Could you check a few things on this model? Use its own coordinates, in mm. A direction names the side the tool comes from. Coordinates: 2 decimals unless noted, no trailing zeros. Loops run counter-clockwise (first coordinate to the right, second up) from the corner with the lowest first, then second, coordinate; pieces in that order, holes last.
1) If I drill on line 1 along Z through (x, y) = (-5, 3.5); line 2 along X through (y, z) = (0.75, 0); line 3 along X through (y, z) = (1, 0.5), over which ranges is the centre line in solid material (lowest first)?
2) Imagine slicing it at C-C on z = 2.25. Please give me the cut outline in (x, y), plus the area to 3 significant figures.
3) For faces 1 (the face through (10, 4, 0)), 2 (the face through (11.5, 5, -9)), 3 (the face through (-11.5, 5, -9)), 4 (the face through (9.75, 2, 0)), which set-ups out of +Z, -Z, +X, -X, +Y, -Y let a thin tool reach every point of the face, with its end or its side?
4) Will these pins go through, and if not, where does the flat tip stop? P1, Ø3, axis at x = 16, z = 0, coming from the +Y side; P2, Ø6, axis at x = -0.5, z = -3.5, coming from the -Y side; P3, Ø1.2, axis at y = 3, z = 0.5, coming from the -X side; P4, Ø2, axis at y = 7.5, z = 3.5, coming from the +X side.
5) Imagine slicing it at A-A on z = 0. Give the number of separate pieces and of enclosed holes in the cut face, plus the area to 3 significant figures.
6) Imagine slicing it at D-D on y = 3.25. Please give me the cut outline in (x, z), plus the area to 4 significant figures.
7) Thinking about a two-plate mould opening in X: for faces 5 (the face through (0, 4, 7.5)), 6 (the face through (-19.5, 1, -9)), 7 (the face through (0, 8, 8)), which applies, released by +X, released by -X, zero draft, split by the parting line, or undercut?
8) Imagine slicing it at B-B on x = -4. Please give me the cut outline in (y, z), plus the area to 3 significant figures.
```python
from build123d import *

# Parameters (mm, degrees)
SKETCH_1_W          = 40
SKETCH_1_H          = 19
EXTRUDE_1_DEPTH     = 8
SKETCH_2_W          = 42
SKETCH_2_H          = 21
SKETCH_2_W_2        = 24
SKETCH_2_H_2        = 19
CUT_EXTRUDE_1_DEPTH = 6
SKETCH_3_W          = 19.5
SKETCH_3_H          = 15
CUT_EXTRUDE_2_DEPTH = 6
SKETCH_5_W          = 17
SKETCH_5_H          = 15
CUT_EXTRUDE_3_DEPTH = 8
SKETCH_6_W          = 15
SKETCH_6_H          = 2.2
CUT_EXTRUDE_4_DEPTH = 1.2
CHAMFER_1_SIZE      = 1.8
CHAMFER_2_SIZE      = 1
CHAMFER_3_SIZE      = 1
SKETCH_7_R          = 1.35
CUT_EXTRUDE_5_DEPTH = 23.940139494


with BuildPart() as part:
    # Эскиз1 → Бобышка-Вытянуть1 (new body)
    with BuildSketch(Plane(origin=(0, 0, 0), x_dir=(1, 0, 0), z_dir=(0, 1, 0))):
        Rectangle(SKETCH_1_W, SKETCH_1_H)
    extrude(amount=EXTRUDE_1_DEPTH)

    # Эскиз2 → Вырез-Вытянуть1 (cut)
    with BuildSketch(Plane(origin=(0, 8, 0), x_dir=(1, 0, 0), z_dir=(0, 1, 0))):
        Rectangle(SKETCH_2_W, SKETCH_2_H)
        Rectangle(SKETCH_2_W_2, SKETCH_2_H_2, mode=Mode.SUBTRACT)
    extrude(amount=-CUT_EXTRUDE_1_DEPTH, mode=Mode.SUBTRACT)

    # Эскиз3 → Вырез-Вытянуть2 (cut)
    with BuildSketch(Plane(origin=(0, 8, 0), x_dir=(1, 0, 0), z_dir=(0, 1, 0))):
        Rectangle(SKETCH_3_W, SKETCH_3_H)
    extrude(amount=-CUT_EXTRUDE_2_DEPTH, mode=Mode.SUBTRACT)

    # Эскиз5 → Вырез-Вытянуть3 (cut)
    with BuildSketch(Plane(origin=(0, 2, 0), x_dir=(1, 0, 0), z_dir=(0, 1, 0))):
        with Locations((1.25, 0)):
            Rectangle(SKETCH_5_W, SKETCH_5_H)
    extrude(amount=-CUT_EXTRUDE_3_DEPTH, mode=Mode.SUBTRACT)

    # Эскиз6 → Вырез-Вытянуть4 (cut)
    with BuildSketch(Plane(origin=(-9.75, 0, 0), x_dir=(0, 0, -1), z_dir=(1, 0, 0))):
        with Locations((0, 5.1)):
            Rectangle(SKETCH_6_W, SKETCH_6_H)
    cut_extrude_4 = extrude(amount=-CUT_EXTRUDE_4_DEPTH, mode=Mode.SUBTRACT)

    # Зеркальное отражение1: Вырез-Вытянуть4 across plane
    add(cut_extrude_4.mirror(Plane(origin=(0, 0, 0), x_dir=(0, 0, 1), z_dir=(1, 0, 0))), mode=Mode.SUBTRACT)

    # Фаска1
    chamfer_1_edges = [part.edges().sort_by_distance(p)[0] for p in [
        (-7.25, 2, 0),
    ]]
    chamfer(chamfer_1_edges, length=CHAMFER_1_SIZE)

    # Фаска2
    chamfer_2_edges = [part.edges().sort_by_distance(p)[0] for p in [
        (-12, 5, -9.5),
        (12, 5, -9.5),
        (12, 5, 9.5),
        (-12, 5, 9.5),
    ]]
    chamfer(chamfer_2_edges, length=CHAMFER_2_SIZE)

    # Фаска3
    chamfer_3_edges = [part.edges().sort_by_distance(p)[0] for p in [
        (-20, 1, -9.5),
        (20, 1, -9.5),
        (20, 1, 9.5),
        (-20, 1, 9.5),
    ]]
    chamfer(chamfer_3_edges, length=CHAMFER_3_SIZE)

    # Эскиз7 → Вырез-Вытянуть5 (cut, through all)
    with BuildSketch(Plane(origin=(0, 2, 0), x_dir=(1, 0, 0), z_dir=(0, 1, 0))):
        with Locations(Location((-16, 0, 0), (0, 0, 270))):
            Circle(SKETCH_7_R)
        with Locations(Location((16, 0, 0), (0, 0, 270))):
            Circle(SKETCH_7_R)
    extrude(amount=-CUT_EXTRUDE_5_DEPTH, mode=Mode.SUBTRACT)


solid = part.part
```
Filled in:
1. line 1: z = -9.5 to -7.5, 7.5 to 9.5
1. line 2: x = -20 to -17.35, -14.65 to -7.8, 9.75 to 14.65, 17.35 to 20
1. line 3: x = -20 to -17.25, -14.75 to -8.05, 9.75 to 14.75, 17.25 to 20
2. outline: (-20, 0) - (-7.25, 0) - (-7.25, 0.2) - (-9.05, 2) - (-9.75, 2) - (-9.75, 4) - (-10.95, 4) - (-10.95, 6.2) - (-9.75, 6.2) - (-9.75, 8) - (-12, 8) - (-12, 2) - (-20, 2) - close; (9.75, 0) - (20, 0) - (20, 2) - (12, 2) - (12, 8) - (9.75, 8) - (9.75, 6.2) - (10.95, 6.2) - (10.95, 4) - (9.75, 4) - close
2. area: 66.1 mm2
3. face 1: none
3. face 2: -Z, +X, +Y
3. face 3: -Z, -X, +Y
3. face 4: +Y, -Y
4. P1: stops at y = 2
4. P2: passes through
4. P3: stops at x = -12
4. P4: stops at x = 12
5. separate pieces: 4
5. enclosed holes: 0
5. area: 55.3 mm2
6. outline: (-12, -8.5) - (-11, -9.5) - (11, -9.5) - (12, -8.5) - (12, 8.5) - (11, 9.5) - (-11, 9.5) - (-12, 8.5) - close; hole (-9.75, -7.5) - (9.75, -7.5) - (9.75, 7.5) - (-9.75, 7.5) - close
6. area: 161.5 mm2
7. face 5: undercut
7. face 6: released by -X
7. face 7: zero draft
8. outline: (0, -9.5) - (8, -9.5) - (8, -7.5) - (0, -7.5) - close; (0, 7.5) - (8, 7.5) - (8, 9.5) - (0, 9.5) - close
8. area: 32.0 mm2
